Can you work these out from the model? Positions are in its coordinate system, mm. Face numbers are marked on the shaded views. A direction names the side the tool comes from. Give positions to 0.01 mm unless a question says otherwise; leave off trailing zeros. Loops run counter-clockwise (first coordinate to the right, second up) from the corner with the lowest first, then second, coordinate; pieces in that order, holes last. Notation, with made-up numbers: (19, 74.25) - (45, 74.25) arc R29 cw to (45, 96.25) - close; hole circle Ø7 at (31, -7.75). An arc over 180 degrees is marked (long way). Use a Markdown table: item, result. Add a question column.
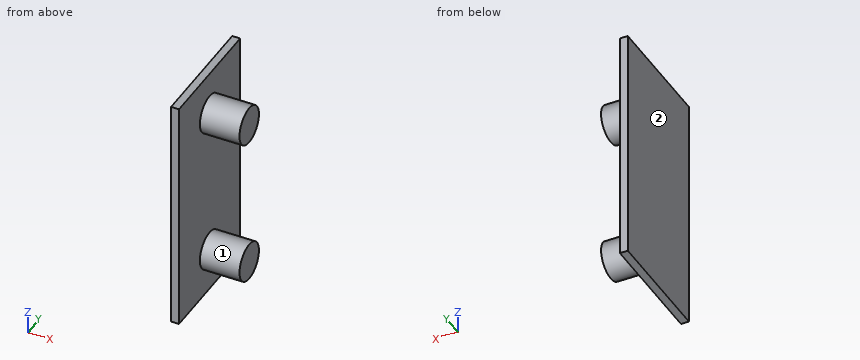
```python
from build123d import *

# Parameters (mm, degrees)
SKETCH2_W           = 60
SKETCH2_H           = 30
SKETCH2_R           = 4.7625
BOSS_EXTRUDE1_DEPTH = 2
BOSS_EXTRUDE2_START = 2
SKETCH2_3_R         = 4.7625
BOSS_EXTRUDE2_DEPTH = 10


with BuildPart() as part:
    # Sketch2 → Boss-Extrude1 (new body)
    # profile 1 of 3: a face of its own
    with BuildSketch(Plane(origin=(0, 0, 0), x_dir=(0, 0, -1), z_dir=(1, 0, 0))):
        Rectangle(SKETCH2_W, SKETCH2_H)
        with Locations((19.05, 0)):
            Circle(SKETCH2_R, mode=Mode.SUBTRACT)
        with Locations((-19.05, 0)):
            Circle(SKETCH2_R, mode=Mode.SUBTRACT)
    # profile 2 of 3: a face of its own
    with BuildSketch(Plane(origin=(0, 0, 0), x_dir=(0, 0, -1), z_dir=(1, 0, 0))):
        with Locations((19.05, 0)):
            Circle(SKETCH2_R)
    # profile 3 of 3: a face of its own
    with BuildSketch(Plane(origin=(0, 0, 0), x_dir=(0, 0, -1), z_dir=(1, 0, 0))):
        with Locations((-19.05, 0)):
            Circle(SKETCH2_R)
    extrude(amount=BOSS_EXTRUDE1_DEPTH)

    # Sketch2<3> → Boss-Extrude2 (add)
    with BuildSketch(Plane(origin=(0, 0, 0), x_dir=(0, 0, -1), z_dir=(1, 0, 0)).offset(BOSS_EXTRUDE2_START)):
        with Locations((-19.05, 0)):
            Circle(SKETCH2_3_R)
        with Locations((19.05, 0)):
            Circle(SKETCH2_3_R)
    extrude(amount=BOSS_EXTRUDE2_DEPTH)


solid = part.part
```
1. On a 3-axis mill with a long thin cutter (end or side, diameter ignored), from which of +Z, -Z, +X, -X, +Y, -Y can I reach the whole of each face in a straight line? I mean the marked faces 1 and 2. Say none if no direction works.
2. Suppose I cut it at A-A (y = 0). List the corners of the cut face in (x, z) for me, and give its area (4 significant figures).
3. Suppose I cut it at D-D (y = 5.75). List the corners of the cut face in (x, z) for me.
4. Will these pins go through, and if not, where does the flat tip stop? P1, Ø1, axis at x = 10.5, y = -2, coming from the -Z side; P2, Ø6, axis at y = -11.5, z = 7.5, coming from the +X side.
5. Please list where these lines run through material, in increasing order: line 1 along X through (y, z) = (-2.5, -10.5); line 2 along Z through (x, y) = (11.75, 2); line 3 along Z through (x, y) = (6, -4). Write a range as [from, to].
6. Suppose I cut it at B-B (z = 19.05). List the corners of the cut face in (x, y) for me.
Results below:
| question | item | result |
|---|---|---|
| 1 | face 1 | +X |
| 1 | face 2 | +Z, -Z, -X, +Y, -Y |
| 2 | outline | (0, -30) - (2, -30) - (2, -23.81) - (12, -23.81) - (12, -14.29) - (2, -14.29) - (2, 14.29) - (12, 14.29) - (12, 23.81) - (2, 23.81) - (2, 30) - (0, 30) - close |
| 2 | area | 310.5 mm² |
| 3 | outline | (0, -30) - (2, -30) - (2, 30) - (0, 30) - close |
| 4 | P1 | z = -23.57 |
| 4 | P2 | x = 2 |
| 5 | line 1 | [0, 2] |
| 5 | line 2 | [-23.37, -14.73], [14.73, 23.37] |
| 5 | line 3 | [-21.63, -16.47], [16.47, 21.63] |
| 6 | outline | (0, -15) - (2, -15) - (2, -4.76) - (12, -4.76) - (12, 4.76) - (2, 4.76) - (2, 15) - (0, 15) - close |
